from build123d import *

# Parameters (mm, degrees)
SM_BASE_FLANGE_1_DEPTH = 3
SKETCH_4_W             = 20
SKETCH_4_H             = 3
EXTRUDE_1_DEPTH        = 2
SKETCH_5_R             = 3
CUT_EXTRUDE_1_DEPTH    = 10


# Sheet-metal steps are written as plain solids
with BuildPart() as part:
    # Sketch 1 → Базовая кромка1 (new body)
    with BuildSketch(Plane.XY):
        with BuildLine():
            Line((-52.715343227, 26.180564784), (241.084656773, 26.180564784))
            ThreePointArc((241.084656773, 26.180564784), (241.862474232, 25.858382243), (242.184656773, 25.080564784))
            Line((242.184656773, 25.080564784), (242.184656773, 1.180564784))
            Line((242.184656773, 1.180564784), (-53.815343227, 1.180564784))
            Line((-53.815343227, 1.180564784), (-53.815343227, 25.080564784))
            ThreePointArc((-53.815343227, 25.080564784), (-53.493160687, 25.858382243), (-52.715343227, 26.180564784))
        make_face()
    extrude(amount=-SM_BASE_FLANGE_1_DEPTH)

    # Эскиз4 → Бобышка-Вытянуть1 (add)
    with BuildSketch(Plane(origin=(0, 26.180564784, 0), x_dir=(1, 0, 0), z_dir=(0, 1, 0))):
        with Locations((-5.815343227, 1.5)):
            Rectangle(SKETCH_4_W, SKETCH_4_H)
        with Locations((194.184656773, 1.5)):
            Rectangle(SKETCH_4_W, SKETCH_4_H)
    extrude(amount=EXTRUDE_1_DEPTH)

    # Эскиз5 → Вырез-Вытянуть1 (cut)
    with BuildSketch(Plane(origin=(0, 0, -3), x_dir=(-1, 0, 0), z_dir=(0, 0, -1))):
        with Locations((-222.184656773, 13.130564784)):
            Circle(SKETCH_5_R)
        with Locations((33.815343227, 13.130564784)):
            Circle(SKETCH_5_R)
    extrude(amount=-CUT_EXTRUDE_1_DEPTH, mode=Mode.SUBTRACT)


solid = part.part
CAD build for the part. Positions are in the model's coordinates, mm. Coordinates: 2 decimals unless noted, no trailing zeros. Write each loop counter-clockwise with the first axis right and the second up, starting at its lowest first coordinate (ties: lowest second). Pieces come first, ordered by that corner, then holes. Notation, with made-up numbers: (81, 66) - (93, 66) arc R21 cw to (93, 82) - close; hole circle Ø10 at (-35.5, -39.75). An arc over 180 degrees is marked (long way). Use a Markdown table: item, result. Add a question column.
Item 1: Drill centre lines: L1, parallel to X at y = 11.25, z = -1.85; L2, parallel to X at y = 12, z = -0.55; L3, parallel to Y at x = 143, z = -2.85. Where is each one in solid material? Low to high. Write a range as from..to.
Item 2: Flat gauge pins, fed straight in: pin 1 (0.6 mm diameter, centred on y = 27.5, z = -1.5, fed in from +X); pin 2 (1.5 mm diameter, centred on x = 224.5, z = -2, fed in from +Y); pin 3 (0.6 mm diameter, centred on y = 27, z = -2, fed in from -X); pin 4 (3.5 mm diameter, centred on x = -33.82, y = 13.13, fed in from +Z). Where does each tip first touch, or does it go through?
Item 3: Mould opens along X. For faces 1 (the face through (96, 15, 0)), 2 (the face through (225.18, 13.26, -1.52)) say: pulls with the +X half, pulls with the -X half, needs draft (parallel to the pull), parting line crosses it, or undercut.
Item 4: Band-saw the part on A-A, the plane z = -1.25. Give the cut face in (x, y).
Item 5: Band-saw the part on B-B, the plane x = 41. Give the cut face in (y, z).
Numbers:
| question | item | result |
|---|---|---|
| 1 | L1 | -53.82..-36.15, -31.48..219.85, 224.52..242.18 |
| 1 | L2 | -53.82..-36.59, -31.04..219.41, 224.96..242.18 |
| 1 | L3 | 1.18..26.18 |
| 2 | pin 1 | x = 204.18 |
| 2 | pin 2 | y = 26.18 |
| 2 | pin 3 | x = -15.82 |
| 2 | pin 4 | through |
| 3 | face 1 | needs draft |
| 3 | face 2 | undercut |
| 4 | outline | (-53.82, 1.18) - (242.18, 1.18) - (242.18, 25.08) arc R1.1 ccw to (241.08, 26.18) - (204.18, 26.18) - (204.18, 28.18) - (184.18, 28.18) - (184.18, 26.18) - (4.18, 26.18) - (4.18, 28.18) - (-15.82, 28.18) - (-15.82, 26.18) - (-52.72, 26.18) arc R1.1 ccw to (-53.82, 25.08) - close; hole circle Ø6 at (-33.82, 13.13); hole circle Ø6 at (222.18, 13.13) |
| 5 | outline | (1.18, -3) - (26.18, -3) - (26.18, 0) - (1.18, 0) - close |
